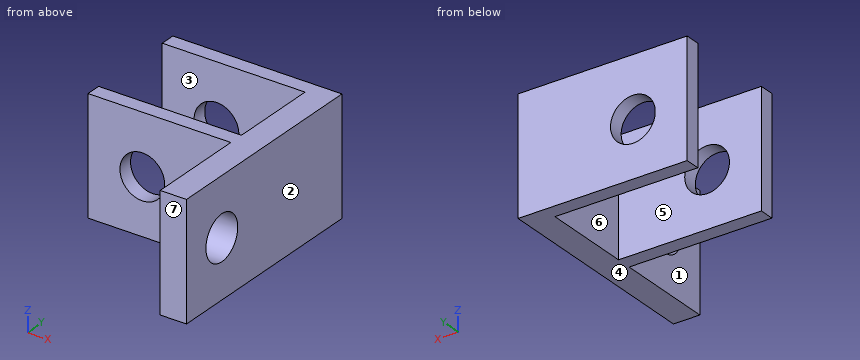
Autodesk Inventor part; units mm, degrees
ref_plane "YZ Plane" through (0, 0, 0) normal (1, 0, 0) x (0, 1, 0)
ref_plane "XZ Plane" through (0, 0, 0) normal (0, 1, 0) x (-1, 0, 0)
ref_plane "XY Plane" through (0, 0, 0) normal (0, 0, 1) x (1, 0, 0)
sketch "Sketch1" plane through (0, 0, 0) normal (1, 0, 0) x (0, 1, 0)
  line L0 (0, 0) -> (12, 0)
  line L1 (12, 0) -> (12, -11.65)
  line L2 (12, -11.65) -> (0, -11.65)
  line L3 (0, -11.65) -> (0, 0)
  dimension "d0" = 12
  dimension "d1" = 11.65
extrude "Extrusion1" add sketch "Sketch1" along normal blind 17
sketch "Sketch3" plane through (0, 0, 0) normal (0, 0, 1) x (1, 0, 0)
  line L0 (-0.6451, 10.5) -> (14.3549, 10.5)
  line L1 (14.3549, 10.5) -> (14.3549, 1.5)
  line L2 (14.3549, 1.5) -> (-0.6451, 1.5)
  line L3 (-0.6451, 1.5) -> (-0.6451, 10.5)
  line L4 (17, 12) -> (17, 0)
  line L5 (0, 12) -> (17, 12)
  point P0 (0, 0)
  point P1 (10, 1.5)
  point P2 (10, 10.5)
  dimension "d7" = 9
  dimension "d8" = 15
  dimension "d10" = 1.5
extrude "Extrusion2" cut sketch "Sketch3" against normal blind 14
sketch "Sketch5" plane through (0, 12, 0) normal (0, 1, 0) x (1, 0, 0)
  circle A0 centre (5.4549, 6.05) radius 2.25
  line L0 (14.3549, 0) -> (14.3549, 11.65)
  line L1 (0, 11.65) -> (17, 11.65)
  point P0 (0, 0)
  point P1 (11.3549, 10)
  point P2 (14.3549, 11.65)
  dimension "d16" = 4.5
  dimension "d17" = 8.9
  dimension "d18" = 5.6
extrude "Extrusion3" cut sketch "Sketch5" against normal blind 14
sketch "Sketch6" plane through (0, 0, -11.65) normal (0, -1, 0) x (1, 0, 0)
  line L0 (14.3549, 11.65) -> (14.3549, 0)
  line L1 (17, 11.65) -> (17, 0)
  line L2 (14.3549, 11.65) -> (17, 11.65)
  line L3 (17, 11.65) -> (17, 0)
  line L4 (17, 0) -> (14.3549, 0)
  line L5 (14.3549, 0) -> (14.3549, 11.65)
  point P0 (0, 11.65)
extrude "Extrusion4" add sketch "Sketch6" along normal blind 10
sketch "Sketch7" plane through (14.3549, 0, -11.65) normal (-1, 0, 0) x (0, 0, 1)
  circle A0 centre (5.825, -5) radius 2.25
  line L0 (11.65, 0) -> (11.65, -10)
  line L1 (11.65, -10) -> (0, -10)
  dimension "d23" = 5.825
  dimension "d24" = 4.5
  dimension "d25" = 5
extrude "Extrusion5" cut sketch "Sketch7" against normal blind 4
properties part number "rodclamp1"
Here's how the part is built. I have some questions about the finished solid (model axes, mm). Face numbers are marked on the shaded views. A direction names the side the tool comes from. Coordinates: 2 decimals unless noted, no trailing zeros. Write each loop counter-clockwise with the first axis right and the second up, starting at its lowest first coordinate (ties: lowest second). Pieces come first, ordered by that corner, then holes.
Item 1: I want a section at A-A on x = 11. Write out the boundary of the cut face in (y, z).
Item 2: Will these pins go through, and if not, where does the flat tip stop? pin 1 (6 mm diameter, centred on y = -4, z = -9.5, fed in from -X); pin 2 (2.5 mm diameter, centred on x = 5.45, z = -6.05, fed in from -Y); pin 3 (6 mm diameter, centred on x = 6.5, z = -6, fed in from -Y).
Item 3: If we mould it in two halves opening along Y, with no side actions, what happens to the marked faces 4, 5, 6 and 7? For each: +Y half, -Y half, draft (parallel to the pull), parting line (faces both ways), or undercut.
Item 4: I want a section at D-D on x = 5.25. Write out the boundary of the cut face in (y, z), and give its area (3 significant figures).
Item 5: On a 3-axis mill with a long thin cutter (end or side, diameter ignored), from which of +Z, -Z, +X, -X, +Y, -Y can I reach the whole of each face in a straight line? I mean the marked faces 1, 2 and 3. Say none if no direction works.
Item 6: If I drill on line 1 (Y direction, x = 9, z = -7.75); line 2 (X direction, y = 1.05, z = -6.05); line 3 (X direction, y = 5.25, z = -4.25), over which ranges is the centre line in solid material (lowest first)?
Item 7: I want a section at C-C on z = -2.25. Write out the boundary of the cut face in (x, y), and give its area (3 significant figures).
Item 8: I want a section at B-B on y = -5. Write out the boundary of the cut face in (x, z) (3 decimals), and give its area (3 significant figures).
Findings below:
1. outline: (0, -11.65) - (1.5, -11.65) - (1.5, 0) - (0, 0) - close; (10.5, -11.65) - (12, -11.65) - (12, 0) - (10.5, 0) - close
2. pin 1: stops at x = 14.35
2. pin 2: passes through
2. pin 3: stops at y = 0
3. face 4: draft
3. face 5: undercut
3. face 6: undercut
3. face 7: -Y half
4. outline: (0, -11.65) - (1.5, -11.65) - (1.5, -8.29) - (0, -8.29) - close; (0, -3.81) - (1.5, -3.81) - (1.5, 0) - (0, 0) - close; (10.5, -11.65) - (12, -11.65) - (12, -8.29) - (10.5, -8.29) - close; (10.5, -3.81) - (12, -3.81) - (12, 0) - (10.5, 0) - close
4. area: 21.5 mm2
5. face 1: +Z, -Z, -X, -Y
5. face 2: +Z, -Z, +X, +Y, -Y
5. face 3: +Z, -Z, -X
6. line 1: y = 0 to 1.5, 10.5 to 12
6. line 2: x = 0 to 3.2, 7.7 to 17
6. line 3: x = 14.35 to 17
7. outline: (0, 0) - (14.35, 0) - (14.35, -10) - (17, -10) - (17, 12) - (0, 12) - (0, 10.5) - (14.35, 10.5) - (14.35, 1.5) - (0, 1.5) - close
7. area: 101 mm2
8. outline: (14.355, -11.65) - (17, -11.65) - (17, -8.075) - (14.355, -8.075) - close; (14.355, -3.575) - (17, -3.575) - (17, 0) - (14.355, 0) - close
8. area: 18.9 mm2
